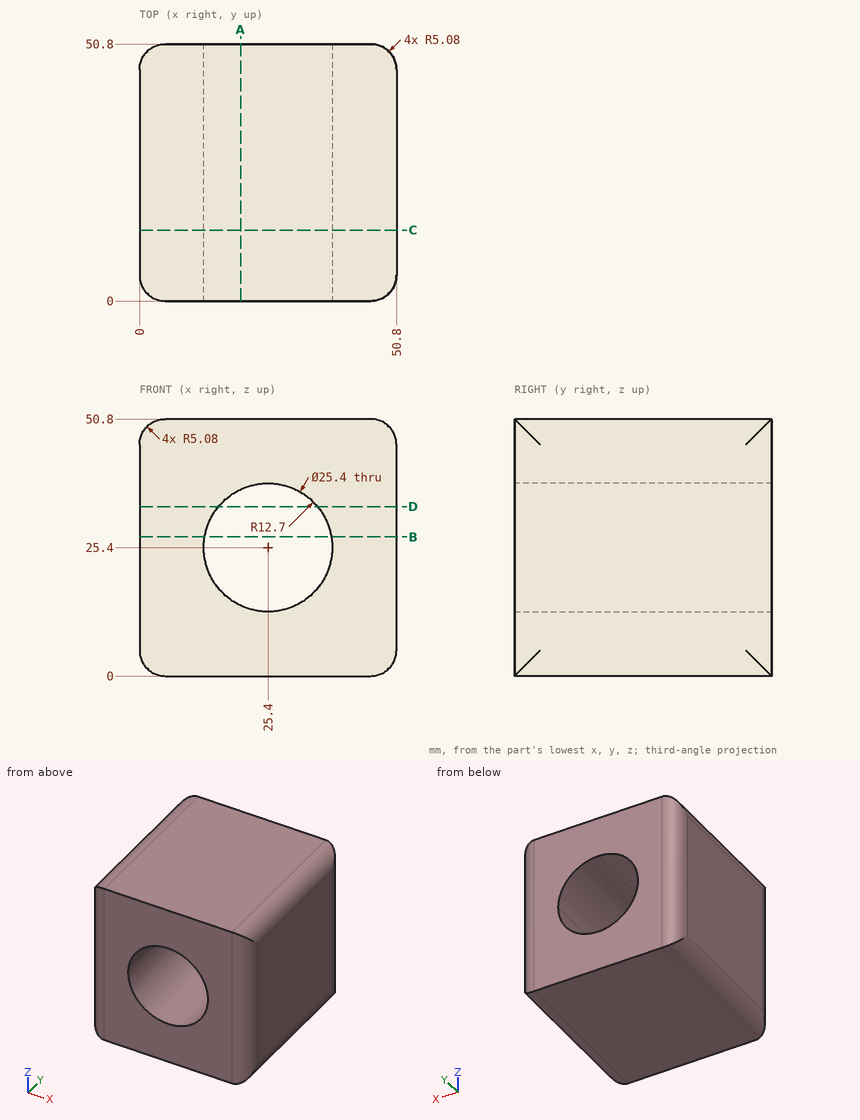
Design review of the part shown in the three views and the two pictorial views. Dimensions are in mm from the part's minimum x, y and z. Round coordinates to 2 decimals unless told otherwise and drop trailing zeros. Order: outer loops, then holes, each group sorted by start corner. A loop starts at its lowest first (then second) coordinate and runs counter-clockwise, first axis right, second up. Notation, with made-up numbers: (21.25, 35) -> (79.25, 35) arc R25 cw to (79.25, 71) -> close; hole circle Ø8 at (-1, -3.5). An arc over 180 degrees is marked (long way). Write item = value, one per line. Start each with the question number.
1) Take a section at B-B on z = 27.5. State the section outline as (x, y) points, plus the area to 3 significant figures.
2) Insertion check: pin 1 (15 mm diameter, centred on x = 25.4, z = 25.4, fed in from +Y). The pin has a flat end and moves straight along its axis. Give the tip position at first contact, or say it passes through.
3) Take a section at A-A on x = 20. State the section outline as (y, z) points.
4) To check wall thickness, follow line 1 (Z direction, x = 25, y = 17); line 2 (Z direction, x = 14.5, y = 5). State the ranges of each line that lie inside material, in increasing order. Write a range as from..to.
5) Take a section at D-D on z = 33.5. State the section outline as (x, y) points.
6) Take a section at C-C on y = 14. State the section outline as (x, z) points, plus the area to 3 significant figures.
Verdict:
q1.outline = (0, 5.08) arc R5.08 ccw to (5.08, 0) -> (12.87, 0) -> (12.87, 50.8) -> (5.08, 50.8) arc R5.08 ccw to (0, 45.72) -> close; (37.93, 0) -> (45.72, 0) arc R5.08 ccw to (50.8, 5.08) -> (50.8, 45.72) arc R5.08 ccw to (45.72, 50.8) -> (37.93, 50.8) -> close
q1.area = 1,290 mm2
q2.pin_1 = through
q3.outline = (0, 0) -> (50.8, 0) -> (50.8, 13.91) -> (0, 13.91) -> close; (0, 36.89) -> (50.8, 36.89) -> (50.8, 50.8) -> (0, 50.8) -> close
q4.line_1 = 0..12.71, 38.09..50.8
q4.line_2 = 0..18.88, 31.92..50.8
q5.outline = (0, 5.08) arc R5.08 ccw to (5.08, 0) -> (15.62, 0) -> (15.62, 50.8) -> (5.08, 50.8) arc R5.08 ccw to (0, 45.72) -> close; (35.18, 0) -> (45.72, 0) arc R5.08 ccw to (50.8, 5.08) -> (50.8, 45.72) arc R5.08 ccw to (45.72, 50.8) -> (35.18, 50.8) -> close
q6.outline = (0, 5.08) arc R5.08 ccw to (5.08, 0) -> (45.72, 0) arc R5.08 ccw to (50.8, 5.08) -> (50.8, 45.72) arc R5.08 ccw to (45.72, 50.8) -> (5.08, 50.8) arc R5.08 ccw to (0, 45.72) -> close; hole circle Ø25.4 at (25.4, 25.4)
q6.area = 2,050 mm2
